Source: CAD feature listing. Evaluate the final solid. Frame: model axes, mm. A direction names the side the tool comes from. Give positions to 0.01 mm unless a question says otherwise; leave off trailing zeros. Answer as a JSON object with one key per item and string values. Group by question number.
Autodesk Inventor part; units mm, degrees
ref_plane "Work Plane3" through (7.5, 0, 0) normal (1, 0, 0) x (0, 1, 0)
ref_plane "XZ Plane" through (0, 0, 0) normal (0, 1, 0) x (-1, 0, 0)
ref_plane "XY Plane" through (0, 0, 0) normal (0, 0, 1) x (1, 0, 0)
sketch "Esboço1" plane through (0, 0, 0) normal (0, 0, 1) x (1, 0, 0)
  circle A0 centre (0, 0) radius 37.5
  circle A1 centre (0, 0) radius 32.5
  circle A2 centre (0, 0) radius 20
  circle A3 centre (20, 0) radius 11
  circle A4 centre (0, 20) radius 11
  circle A5 centre (-20, 0) radius 11
  circle A6 centre (0, -20) radius 11
  circle A7 centre (0, 0) radius 7.5
  circle A8 centre (0, 0) radius 3
  dimension "d2" = 40
  dimension "d17" = 1
  dimension "d0" = 75
  dimension "d1" = 65
  dimension "d3" = 22
  dimension "d6" = 360
  dimension "d8" = 15
  dimension "d9" = 6
extrude "Extrusão1" add sketch "Esboço1" along normal mid plane 10 contours A0
extrude "Extrusão2" add sketch "Esboço1" along normal mid plane 4 contours A1 | A3 A2 A6 A5 A4
extrude "Extrusão3" add sketch "Esboço1" along normal mid plane 10 contours A7
fillet "Arredondamento1" radius 2 2 edges at (-37.5, 0, 5) (-37.5, 0, -5)
fillet "Arredondamento2" radius 1 2 edges at (-7.5, 0, 5) (-7.5, 0, -5)
sketch "Esboço2" plane through (0, 0, 2) normal (0, 0, 1) x (1, 0, 0)
  point P0 (0, 0)
  dimension "d17" = 1
ref_plane "Work Plane3" through (7.5, 0, 0) normal (1, 0, 0) x (0, 1, 0)
sketch "Sketch8" plane through (7.5, 0, 0) normal (1, 0, 0) x (0, 1, 0)
  line L0 (-7.5, -5) -> (7.5, -5)
  line L1 (7.5, -2) -> (-7.5, -2)
  line L2 (0, -2) -> (0, -4.5)
  circle A0 centre (0, -3.25) radius 1.25
  point P0 (0, 0)
  dimension "d17" = 1
  dimension "d34" = 2.5
sketch "Sketch9" plane through (0, 0, 0) normal (0, 1, 0) x (-1, 0, 0)
  line L0 (-3.4847, 0.1554) -> (-11.509, -4.1521)
  line L1 (-3, 5) -> (-3, -5)
  line L2 (-2.8935, -0.9459) -> (-10.9178, -5.2534)
  line L3 (-10.9178, -5.2534) -> (-11.509, -4.1521)
  line L4 (-3.4847, 0.1554) -> (-2.8935, -0.9459)
  point P0 (0, 0)
  point P1 (-7.5, -2)
  point P2 (-3, -1.0031)
  point P3 (-3, -0.7476)
  dimension "d40" = 1.25
revolve "Revolution1" cut sketch "Sketch9" angle 360 about axis through (2.8935, 0, -0.9459) along (0.8810792, 0, -0.4729688) contours L4 L1 L2 L3 L0
thread "Thread1"
properties part number "fly_wheel" material "Aluminum 6061-AHC"
(1) Pull-direction query (Z, two-part tool) for faces 4 (the cylindrical face through (-9.839, 4.213, -0.028)), 5 (the flat face through (0, 8, 2)), 6 (the cylindrical face through (4.803, -0.055, -3.388)), 7 (the flat face through (3, -1, -5)); classes: pulls with the +Z half, pulls with the -Z half, needs draft (parallel to the pull), parting line crosses it, or undercut.
(2) Contact query for flat-ended pins moving along their axis: pin 1 Ø5 at (y, z) = (16.5, 0) entering from -X; pin 2 Ø6 at (y, z) = (-15, 0.5) entering from +X; pin 3 Ø4 at (x, z) = (-16, -2.5) entering from +Y. Output: stop coordinate, or through.
(3) Ray query, L1, parallel to Y at x = 0, z = -3.1; L2, parallel to Y at x = 0, z = 0.1; L3, parallel to X at y = -5.5, z = -2.75. Return the intervals inside material, ascending. Write a range as [from, to].
(4) Access query for faces 1 (the cylindrical face through (31, -9.76, 3.48)), 2 (the cylindrical face through (-2.38, 30.74, -0.03)), 3 (the cylindrical face through (31, 9.76, -3.48)). Directions: +Z, -Z, +X, -X, +Y, -Y. A direction counts if a zero-diameter tool reaches every point of the face in a straight line with its end or side. Return the directions, or none.
(5) Section A-A, the plane x = 0. State how many separate pieces and enclosed holes the cut face has, plus the area to 3 significant figures.
Reported:
{
 "1": {"face 4": "needs draft", "face 5": "pulls with the +Z half", "face 6": "undercut", "face 7": "pulls with the -Z half"},
 "2": {"pin 1": "stops at x = -34.79", "pin 2": "stops at x = 35.53", "pin 3": "stops at y = 34.79"},
 "3": {"L1": "y = [-37.5, -32.5], [-7.5, -3], [3, 7.5], [32.5, 37.5]", "L2": "y = [-37.5, -31], [-9, -3], [3, 9], [31, 37.5]", "L3": "x = [-37.09, -32.03], [-5.1, 5.1], [32.03, 37.09]"},
 "4": {"face 1": "+Z", "face 2": "+Z, -Z", "face 3": "-Z"},
 "5": {"separate pieces": "4", "enclosed holes": "0", "area": "210 mm2"}
}
